from build123d import *

# Parameters (mm, degrees)
SKETCH1_W           = 12.5
SKETCH1_H           = 50
BOSS_EXTRUDE1_DEPTH = 50
BOSS_EXTRUDE2_DEPTH = 15
SKETCH3_R           = 15
CUT_EXTRUDE3_DEPTH  = 150
SKETCH3_3_R         = 20
SKETCH3_3_R_2       = 15
CUT_EXTRUDE4_DEPTH  = 25
CUT_EXTRUDE7_DEPTH  = 20
CUT_EXTRUDE8_DEPTH  = 20


with BuildPart() as part:
    # Sketch1 → Boss-Extrude1 (new body)
    with BuildSketch(Plane.XY):
        Polygon((-26.239919355, -7.714717742), (-51.239919355, -7.714717742), (-51.239919355, -32.714717742), (48.760080645, -32.714717742), (48.760080645, -7.714717742), (23.760080645, -7.714717742), (23.760080645, 17.285282258), (-26.239919355, 17.285282258), align=None)
        with Locations((-44.989919355, 17.285282258)):
            Rectangle(SKETCH1_W, SKETCH1_H)
        with Locations((42.510080645, 17.285282258)):
            Rectangle(SKETCH1_W, SKETCH1_H)
    extrude(amount=BOSS_EXTRUDE1_DEPTH)

    # Sketch1_3 → Boss-Extrude2 (add)
    with BuildSketch(Plane.XY):
        Polygon((-38.739919355, 42.285282258), (-38.739919355, -7.714717742), (-26.239919355, -7.714717742), (-26.239919355, 17.285282258), (23.760080645, 17.285282258), (23.760080645, -7.714717742), (36.260080645, -7.714717742), (36.260080645, 42.285282258), (48.760080645, 42.285282258), (48.760080645, 67.285282258), (23.760080645, 67.285282258), (23.760080645, 42.285282258), (-26.239919355, 42.285282258), (-26.239919355, 67.285282258), (-51.239919355, 67.285282258), (-51.239919355, 42.285282258), align=None)
    extrude(amount=BOSS_EXTRUDE2_DEPTH)

    # Sketch3 → Cut-Extrude3 (cut)
    with BuildSketch(Plane(origin=(0, 17.285282258, 0), x_dir=(1, 0, 0), z_dir=(0, 1, 0))):
        with Locations((-1.239919355, -50)):
            Circle(SKETCH3_R)
    extrude(amount=-CUT_EXTRUDE3_DEPTH, mode=Mode.SUBTRACT)

    # Sketch3_3 → Cut-Extrude4 (cut)
    with BuildSketch(Plane(origin=(0, 17.285282258, 0), x_dir=(1, 0, 0), z_dir=(0, 1, 0))):
        with Locations((-1.239919355, -50)):
            Circle(SKETCH3_3_R)
        with Locations((-1.239919355, -50)):
            Circle(SKETCH3_3_R_2, mode=Mode.SUBTRACT)
    extrude(amount=-CUT_EXTRUDE4_DEPTH, mode=Mode.SUBTRACT)

    # Sketch6 → Cut-Extrude7 (cut)
    with BuildSketch(Plane(origin=(48.760080645, 0, 0), x_dir=(0, 0, -1), z_dir=(1, 0, 0))):
        Polygon((-50, 42.285282258), (-50, -7.714717742), (-15, 42.285282258), align=None)
    extrude(amount=-CUT_EXTRUDE7_DEPTH, mode=Mode.SUBTRACT)

    # Sketch7 → Cut-Extrude8 (cut)
    with BuildSketch(Plane(origin=(-38.739919355, 0, 0), x_dir=(0, 0, -1), z_dir=(1, 0, 0))):
        Polygon((-50, -7.714717742), (-15, 42.285282258), (-50, 42.285282258), align=None)
    extrude(amount=-CUT_EXTRUDE8_DEPTH, mode=Mode.SUBTRACT)


solid = part.part
Source: CAD feature listing. Evaluate the final solid. Frame: model axes, mm. A direction names the side the tool comes from. Round coordinates to 2 decimals unless told otherwise and drop trailing zeros. Loops run counter-clockwise (first coordinate to the right, second up) from the corner with the lowest first, then second, coordinate; pieces in that order, holes last. Notation, with made-up numbers: (-20, 18) - (-9, 18) arc R25 cw to (-9, 35) - close; hole circle Ø11 at (73.25, 87.25). An arc over 180 degrees is marked (long way). Write item = value, one per line. Start each with the question number.
(1) Pin query (flat end, axial travel): pin 1 (3 mm diameter, centred on x = 20, z = 7.5, fed in from +Y); pin 2 (6 mm diameter, centred on x = 4.5, z = 36, fed in from +Y); pin 3 (2 mm diameter, centred on x = -1.5, y = -19.5, fed in from +Z). Return the tip coordinate at first contact, or that it passes through.
(2) Ray query, line 1 along X through (y, z) = (5.5, 24); line 2 along X through (y, z) = (47, 7); line 3 along Z through (x, y) = (-13, 24). Return the intervals inside material, ascending. Write a range as from..to.
(3) Section query B-B, the plane z = 42.5. Output: boundary loops of the cut face in (x, y).
(4) Section query C-C, the plane z = 5.5. Output: boundary loops of the cut face in (x, y), plus the area to 3 significant figures.
(5) Section query D-D, the plane x = -43. Output: boundary loops of the cut face in (y, z).
(6) Set-up query: faces 4 (the face through (-26.24, 55, 7)), 5 (the face through (-30, -18, 50)), 6 (the face through (-1, 5, 30)), 7 (the face through (42.598, 16.935, 32.745)), 8 (the face through (48.76, 5, 19)). Return all of +Z, -Z, +X, -X, +Y, -Y with unobstructed straight access to the full face (end or side cutting, diameter ignored); none if empty.
(7) Section query A-A, the plane y = 50.5. Output: boundary loops of the cut face in (x, z), plus the area to 3 significant figures.
(8) Pull-direction query (X, two-part tool) for faces 1 (the face through (-51.24, 7, 19)), 2 (the face through (36, 67.285, 7)), 3 (the face through (23.76, 5, 32)); classes: +X half, -X half, draft (parallel to the pull), parting line (faces both ways), or undercut.
Conclusion:
q1.pin_1 = 42.29
q1.pin_2 = -7.71
q1.pin_3 = 35.05
q2.line_1 = -51.24..-38.74, -26.24..23.76, 36.26..48.76
q2.line_2 = -51.24..-26.24, 23.76..48.76
q2.line_3 = 0..15
q3.outline = (-51.24, -32.71) - (-14.23, -32.71) - (-14.23, -7.71) - (-19.78, -7.71) - (-19.78, 17.29) - (-26.24, 17.29) - (-26.24, -7.71) - (-38.74, -7.71) - (-38.74, 3) - (-51.24, 3) - close; (11.75, -32.71) - (48.76, -32.71) - (48.76, 3) - (36.26, 3) - (36.26, -7.71) - (23.76, -7.71) - (23.76, 17.29) - (17.3, 17.29) - (17.3, -7.71) - (11.75, -7.71) - close
q4.outline = (-51.24, -32.71) - (48.76, -32.71) - (48.76, 67.29) - (23.76, 67.29) - (23.76, 42.29) - (-26.24, 42.29) - (-26.24, 67.29) - (-51.24, 67.29) - close
q4.area = 8,750 mm2
q5.outline = (-32.71, 0) - (67.29, 0) - (67.29, 15) - (42.29, 15) - (-7.71, 50) - (-32.71, 50) - close
q6.face_4 = +Z, -Z, +Y
q6.face_5 = +Z, +X, -X, +Y, -Y
q6.face_6 = +Z, +Y
q6.face_7 = +Z, +X, +Y
q6.face_8 = +Z, -Z, +X, +Y, -Y
q7.outline = (-51.24, 0) - (-26.24, 0) - (-26.24, 15) - (-51.24, 15) - close; (23.76, 0) - (48.76, 0) - (48.76, 15) - (23.76, 15) - close
q7.area = 750 mm2
q8.face_1 = -X half
q8.face_2 = draft
q8.face_3 = undercut
